Geometry check sheet. Reference: the model listing, model coordinates, mm. A direction names the side the tool comes from. Give positions to 0.01 mm unless a question says otherwise; leave off trailing zeros. Loops run counter-clockwise (first coordinate to the right, second up) from the corner with the lowest first, then second, coordinate; pieces in that order, holes last. Notation, with made-up numbers: (70, 35.25) -> (77, 35.25) arc R37 ccw to (77, 71.25) -> close; hole circle Ø7 at (-4.5, 8). An arc over 180 degrees is marked (long way). One line per item, written item: value. Start each with the question number.
(1) Scan lines: line 1 along X through (y, z) = (9.5, 0); line 2 along Y through (x, z) = (-9.5, -31); line 3 along X through (y, z) = (6, 0.5). Record each from-to range of solid material in increasing order. Write a range as from..to.
(2) Gauge pin test, flat ends, axial feed: pin 1 Ø8 at (y, z) = (4, -22) entering from -X; pin 2 Ø4 at (x, z) = (15.5, -11) entering from +Y; pin 3 Ø8 at (y, z) = (3.5, -21) entering from +X; pin 4 Ø8 at (x, z) = (24.5, -7) entering from +Y. Record the tip position at first contact, or that the pin passes through.
(3) Sectioned sample at D-D, the plane y = 16. Record the cut outline in (x, z), then the cut area to 3 significant figures.
(4) Sectioned sample at C-C, the plane x = 0. Record the cut outline in (y, z), then the cut area to 3 significant figures.
(5) Sectioned sample at A-A, the plane y = 20. Record the cut outline in (x, z).
(6) Tool access check on faces 5 (the face through (7, 17.5, 30)), 6 (the face through (-1, 18, -31.35)), 7 (the face through (10, 20, 30)), 8 (the face through (5, 18, -30)). Record the directions out of +Z, -Z, +X, -X, +Y, -Y that give a thin tool (end or side, any length) a straight path to the whole face; none if there is none.
(7) Sectioned sample at B-B, the plane z = 0. Record the cut outline in (x, y).
(8) Draft check along X on faces 1 (the face through (27.85, 18, -1)), 2 (the face through (-30, 18, -5)), 3 (the face through (-19.38, -1.52, 4.3)), 4 (the face through (-10, 20, -30)). Enter one of: pulls with the +X half, pulls with the -X half, needs draft (parallel to the pull), parting line crosses it, or undercut.
from build123d import *

# Parameters (mm, degrees)
SKETCH1_R           = 33.6
SKETCH1_R_2         = 25.6
BOSS_EXTRUDE1_DEPTH = 13
SKETCH2_W           = 10
SKETCH2_H           = 3.5
BOSS_EXTRUDE2_DEPTH = 10
BOSS_EXTRUDE3_START = 3
SKETCH3_R           = 33.6
SKETCH3_R_2         = 19.85
BOSS_EXTRUDE3_DEPTH = 3
SKETCH4_W           = 15
SKETCH4_H           = 5.5
BOSS_EXTRUDE4_DEPTH = 3.5
CIRPATTERN1_COUNT   = 4
FILLET1_R           = 10


with BuildPart() as part:
    # Sketch1 → Boss-Extrude1 (new body)
    with BuildSketch(Plane(origin=(0, 0, 0), x_dir=(1, 0, 0), z_dir=(0, 1, 0))):
        with Locations(Location((0, 0, 0), (0, 0, 90))):
            Circle(SKETCH1_R)
        with Locations(Location((0, 0, 0), (0, 0, 90))):
            Circle(SKETCH1_R_2, mode=Mode.SUBTRACT)
    extrude(amount=BOSS_EXTRUDE1_DEPTH)

    # Sketch2 → Boss-Extrude2 (add)
    with BuildSketch(Plane(origin=(0, 13, 0), x_dir=(1, 0, 0), z_dir=(0, 1, 0))):
        with Locations((0, -29.6)):
            Rectangle(SKETCH2_W, SKETCH2_H)
    boss_extrude2 = extrude(amount=BOSS_EXTRUDE2_DEPTH)

    # Sketch3 → Boss-Extrude3 (add)
    with BuildSketch(Plane.XZ.offset(BOSS_EXTRUDE3_START)):
        with Locations(Location((0, 0, 0), (0, 0, 270))):
            Circle(SKETCH3_R)
        with Locations(Location((0, 0, 0), (0, 0, 270))):
            Circle(SKETCH3_R_2, mode=Mode.SUBTRACT)
    extrude(amount=-BOSS_EXTRUDE3_DEPTH)

    # Sketch4 → Boss-Extrude4 (add)
    with BuildSketch(Plane.XY.offset(31.35)):
        with Locations((2.5, 20.25)):
            Rectangle(SKETCH4_W, SKETCH4_H)
    boss_extrude4 = extrude(amount=-BOSS_EXTRUDE4_DEPTH)

    # CirPattern1: Boss-Extrude2, Boss-Extrude4 ×4 about axis
    cirpattern1_axis = Axis((0, 0, 0), (0, 1, 0))
    add([boss_extrude2.rotate(cirpattern1_axis, i * 360 / CIRPATTERN1_COUNT) for i in range(1, CIRPATTERN1_COUNT)])
    add([boss_extrude4.rotate(cirpattern1_axis, i * 360 / CIRPATTERN1_COUNT) for i in range(1, CIRPATTERN1_COUNT)])

    # Fillet1
    fillet1_edges = [part.edges().sort_by_distance(p)[0] for p in [
        (0, -3, 33.6),
    ]]
    fillet(fillet1_edges, radius=FILLET1_R)


solid = part.part
Calculated:
1. line 1: x = -33.6..-25.6, 25.6..33.6
1. line 2: y = 2.29..13, 17.5..23
1. line 3: x = -33.55..-25.6, 25.6..33.55
2. pin 1: stops at x = -28.06
2. pin 2: stops at y = 0
2. pin 3: stops at x = 28.57
2. pin 4: stops at y = 23
3. outline: (-31.35, -5) -> (-27.85, -5) -> (-27.85, 5) -> (-31.35, 5) -> close; (-5, -31.35) -> (5, -31.35) -> (5, -27.85) -> (-5, -27.85) -> close; (-5, 27.85) -> (5, 27.85) -> (5, 31.35) -> (-5, 31.35) -> close; (27.85, -5) -> (31.35, -5) -> (31.35, 5) -> (27.85, 5) -> close
3. area: 140 mm2
4. outline: (-3, -23.6) arc R10 ccw to (7, -33.6) -> (13, -33.6) -> (13, -31.35) -> (23, -31.35) -> (23, -27.85) -> (13, -27.85) -> (13, -25.6) -> (0, -25.6) -> (0, -19.85) -> (-3, -19.85) -> close; (-3, 19.85) -> (0, 19.85) -> (0, 25.6) -> (13, 25.6) -> (13, 27.85) -> (23, 27.85) -> (23, 31.35) -> (13, 31.35) -> (13, 33.6) -> (7, 33.6) arc R10 ccw to (-3, 23.6) -> close
4. area: 318 mm2
5. outline: (-31.35, -5) -> (-27.85, -5) -> (-27.85, 10) -> (-31.35, 10) -> close; (-10, -31.35) -> (5, -31.35) -> (5, -27.85) -> (-10, -27.85) -> close; (-5, 27.85) -> (10, 27.85) -> (10, 31.35) -> (-5, 31.35) -> close; (27.85, -10) -> (31.35, -10) -> (31.35, 5) -> (27.85, 5) -> close
6. face 5: +Z, -Z, +X
6. face 6: -Z, +X, -X, +Y
6. face 7: +Z, -Z, +X, +Y
6. face 8: -Z, +X, +Y
7. outline: (-33.6, 7) arc R10 ccw to (-23.6, -3) -> (-19.85, -3) -> (-19.85, 0) -> (-25.6, 0) -> (-25.6, 13) -> (-27.85, 13) -> (-27.85, 23) -> (-31.35, 23) -> (-31.35, 13) -> (-33.6, 13) -> close; (19.85, -3) -> (23.6, -3) arc R10 ccw to (33.6, 7) -> (33.6, 13) -> (31.35, 13) -> (31.35, 23) -> (27.85, 23) -> (27.85, 13) -> (25.6, 13) -> (25.6, 0) -> (19.85, 0) -> close
8. face 1: undercut
8. face 2: needs draft
8. face 3: undercut
8. face 4: pulls with the -X half
